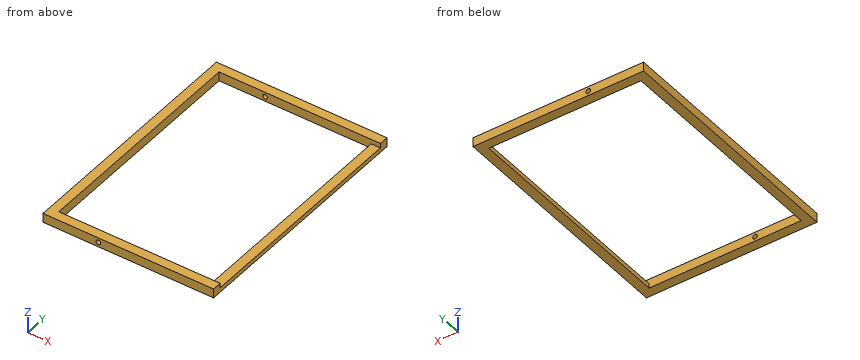
```python
from build123d import *

# Parameters (mm, degrees)
F1_DEPTH = 25.4
F0_W     = 25.4
F0_H     = 619.125
F2_DEPTH = 12.7
F3_R     = 6.35
F4_DEPTH = 762


with BuildPart() as f1:
    # F0 (on Top) → F1 (new body)
    with BuildSketch(Plane.XY):
        Polygon((234.95, 334.9625), (-234.95, 334.9625), (-234.95, -334.9625), (234.95, -334.9625), (234.95, -309.5625), (209.55, -309.5625), (-209.55, -309.5625), (-209.55, 309.5625), (209.55, 309.5625), (234.95, 309.5625), align=None)
    extrude(amount=F1_DEPTH)

    # F0 (on Top) → F2 (join)
    with BuildSketch(Plane.XY):
        with Locations((222.25, 0)):
            Rectangle(F0_W, F0_H)
    extrude(amount=F2_DEPTH)

    # F3 (on face) → F4 (cut)
    with BuildSketch(Plane.XZ.offset(334.9625)):
        with Locations((-82.55, 12.7)):
            Circle(F3_R)
    extrude(amount=-F4_DEPTH, mode=Mode.SUBTRACT)


solid = f1.part
```
Geometry check sheet. Reference: the model listing, model coordinates, mm. Round coordinates to 2 decimals unless told otherwise and drop trailing zeros. Order: outer loops, then holes, each group sorted by start corner. A loop starts at its lowest first (then second) coordinate and runs counter-clockwise, first axis right, second up. Notation, with made-up numbers: (-16, 59.25) - (20, 59.25) arc R13 cw to (20, 73.25) - close; hole circle Ø7 at (-36, -14.5). An arc over 180 degrees is marked (long way). Use a Markdown table: item, result. Add a question column.
1) Section check A-A (y = -2). Record the cut outline in (x, z).
2) Gauge pin test, flat end, axial feed: P1, Ø12.5, axis at x = 226.5, y = -11.5, coming from the +Z side. Record the tip position at first contact, or that the pin passes through.
3) Thickness scan on line 1 along Z through (x, y) = (-82.55, 322.25); line 2 along Y through (x, z) = (-19, 23.75); line 3 along X through (y, z) = (99.5, 12.5). Record the ranges inside material, lowest first.
4) Section check B-B (x = 73). Record the cut outline in (y, z).
Established:
| question | item | result |
|---|---|---|
| 1 | outline | (-234.95, 0) - (-209.55, 0) - (-209.55, 25.4) - (-234.95, 25.4) - close; (209.55, 0) - (234.95, 0) - (234.95, 12.7) - (209.55, 12.7) - close |
| 2 | P1 | z = 12.7 |
| 3 | line 1 | 0 to 6.35, 19.05 to 25.4 |
| 3 | line 2 | -334.96 to -309.56, 309.56 to 334.96 |
| 3 | line 3 | -234.95 to -209.55, 209.55 to 234.95 |
| 4 | outline | (-334.96, 0) - (-309.56, 0) - (-309.56, 25.4) - (-334.96, 25.4) - close; (309.56, 0) - (334.96, 0) - (334.96, 25.4) - (309.56, 25.4) - close |
